```python
from build123d import *

# Parameters (mm, degrees)
SKETCH011_W     = 59.6
SKETCH011_H     = 44
SKETCH011_R     = 1.65
PAD006_DEPTH    = 3
CHAMFER003_SIZE = 1.85
SKETCH012_W     = 3
SKETCH012_H     = 44
PAD007_DEPTH    = 19
POCKET005_DEPTH = 59.601
FILLET_R        = 1.5
FILLET001_R     = 6.2


with BuildPart() as part:
    # Sketch011 → Pad006 (new body)
    with BuildSketch(Plane.YZ):
        with Locations((-29.8, 22)):
            Rectangle(SKETCH011_W, SKETCH011_H)
        with Locations((-49.6, 34.5)):
            Circle(SKETCH011_R, mode=Mode.SUBTRACT)
        with Locations((-19.6, 34.5)):
            Circle(SKETCH011_R, mode=Mode.SUBTRACT)
        with Locations((-49.6, 9.5)):
            Circle(SKETCH011_R, mode=Mode.SUBTRACT)
        with Locations((-19.6, 9.5)):
            Circle(SKETCH011_R, mode=Mode.SUBTRACT)
    extrude(amount=PAD006_DEPTH)

    # Chamfer003
    chamfer003_edges = [part.edges().sort_by_distance(p)[0] for p in [
        (3, -51.25, 34.5),
        (3, -21.25, 34.5),
        (3, -51.25, 9.5),
        (3, -21.25, 9.5),
    ]]
    chamfer(chamfer003_edges, length=CHAMFER003_SIZE)

    # Sketch012 (on Face4 of Chamfer003) → Pad007 (join)
    with BuildSketch(Plane.YZ.offset(3)):
        with Locations((-1.5, 22)):
            Rectangle(SKETCH012_W, SKETCH012_H)
    extrude(amount=PAD007_DEPTH)

    # Sketch013 (on Face16 of Pad007) → Pocket005 (cut, through all)
    with BuildSketch(Plane.ZX):
        with BuildLine():
            ThreePointArc((9.375, 14.7625), (6.125, 18.0125), (2.875, 14.7625))
            Line((2.875, 14.7625), (2.875, 11.7625))
            ThreePointArc((2.875, 11.7625), (6.125, 8.5125), (9.375, 11.7625))
            Line((9.375, 14.7625), (9.375, 11.7625))
        make_face()
        with BuildLine():
            ThreePointArc((41.125, 14.7625), (37.875, 18.0125), (34.625, 14.7625))
            Line((34.625, 14.7625), (34.625, 11.7625))
            ThreePointArc((34.625, 11.7625), (37.875, 8.5125), (41.125, 11.7625))
            Line((41.125, 14.7625), (41.125, 11.7625))
        make_face()
    extrude(amount=-POCKET005_DEPTH, mode=Mode.SUBTRACT)

    # Fillet
    fillet_edges = [part.edges().sort_by_distance(p)[0] for p in [
        (3, -3, 22),
    ]]
    fillet(fillet_edges, radius=FILLET_R)

    # Fillet001
    fillet001_edges = [part.edges().sort_by_distance(p)[0] for p in [
        (22, -1.5, 44),
        (22, -1.5, 0),
    ]]
    fillet(fillet001_edges, radius=FILLET001_R)


solid = part.part
```
Source: CAD feature listing. Evaluate the final solid. Frame: model axes, mm. A direction names the side the tool comes from. Coordinates: 2 decimals unless noted, no trailing zeros. Loops run counter-clockwise (first coordinate to the right, second up) from the corner with the lowest first, then second, coordinate; pieces in that order, holes last. Notation, with made-up numbers: M 46.25,6 L 93.25,6 A35 cw 93.25,42 Z; hole C 31,37 d5. An arc over 180 degrees is marked long. Use a Markdown table: item, result. Add a question column.
Q1. Material intervals for L1, parallel to Z at x = 0.7, y = -49.6; L2, parallel to X at y = -8, z = 33; L3, parallel to Y at x = 18.5, z = 24, sorted ascending.
Q2. First-contact query: pin 1 (8 mm diameter, centred on y = -20, z = 5.5, fed in from +X); pin 2 (1.5 mm diameter, centred on x = 19.5, z = 24.5, fed in from -Y); pin 3 (4.5 mm diameter, centred on y = -19.6, z = 34.5, fed in from +X). Flat tips, straight axial feed; report the tip coordinate or a pass-through.
Q3. Draft query along Y for faces 3 (the cylindrical face through (0.57, -18.71, 35.89)), 4 (the cylindrical face through (3.45, -3.43, 22.31)), 5 (the flat face through (3, -32, 22)). Return one class per face: pulls with the +Y half, pulls with the -Y half, needs draft (parallel to the pull), parting line crosses it, or undercut.
Q4. Section query D-D, the plane y = -36. Return loops of the section in (x, z), and give its area (3 significant figures).
Q5. Section query B-B, the plane z = 18. Return loops of the section in (x, y).
Q6. Access query for faces 1 (the flat face through (0, -30, 22)), 2 (the flat face through (13, -1, 2.875)). Directions: +Z, -Z, +X, -X, +Y, -Y. A direction counts if a zero-diameter tool reaches every point of the face in a straight line with its end or side. Return the directions, or none.
Q7. Section query C-C, the plane x = 7.5. Return loops of the section in (y, z), and give its area (3 significant figures).
Q8. Section query A-A, the plane y = -49.6. Return loops of the section in (x, z), and give its area (3 significant figures).
Result:
| question | item | result |
|---|---|---|
| 1 | L1 | z = 0 to 7.85, 11.15 to 32.85, 36.15 to 44 |
| 1 | L2 | x = 0 to 3 |
| 1 | L3 | y = -3 to 0 |
| 2 | pin 1 | stops at x = 3 |
| 2 | pin 2 | stops at y = -3 |
| 2 | pin 3 | stops at x = 1.75 |
| 3 | face 3 | undercut |
| 3 | face 4 | pulls with the -Y half |
| 3 | face 5 | needs draft |
| 4 | outline | M 0,0 L 3,0 L 3,44 L 0,44 Z |
| 4 | area | 132 mm2 |
| 5 | outline | M 0,-59.6 L 3,-59.6 L 3,-4.5 A1.5 cw 4.5,-3 L 22,-3 L 22,0 L 0,0 Z |
| 6 | face 1 | +Z, -Z, -X, +Y, -Y |
| 6 | face 2 | +Y, -Y |
| 7 | outline | M -3,0 L 0,0 L 0,44 L -3,44 Z |
| 7 | area | 132 mm2 |
| 8 | outline | M 0,0 L 3,0 L 3,6 L 1.15,7.85 L 0,7.85 Z; M 0,11.15 L 1.15,11.15 L 3,13 L 3,31 L 1.15,32.85 L 0,32.85 Z; M 0,36.15 L 1.15,36.15 L 3,38 L 3,44 L 0,44 Z |
| 8 | area | 105 mm2 |
